```python
from build123d import *

# Parameters (mm, degrees)
F0_R     = 6
F1_DEPTH = 23
F2_SIZE  = 0.5
F3_R     = 1.5
F4_DEPTH = 12.5
F5_R     = 2
F6_DEPTH = 10
F7_SIZE  = 0.25


with BuildPart() as f1:
    # F0 (on Front) → F1 (new body)
    with BuildSketch(Plane.XZ):
        Circle(F0_R)
    extrude(amount=F1_DEPTH)

    # F2
    f2_edges = [f1.edges().sort_by_distance(p)[0] for p in [
        (-6, -23, 0),
        (-6, 0, 0),
    ]]
    chamfer(f2_edges, length=F2_SIZE)

    # F3 (on Right) → F4 (cut, symmetric)
    with BuildSketch(Plane.YZ):
        with Locations((-18, 0)):
            Circle(F3_R)
    extrude(amount=F4_DEPTH, both=True, mode=Mode.SUBTRACT)

    # F5 (on face) → F6 (join)
    with BuildSketch(Plane(origin=(0, 0, 0), x_dir=(-1, 0, 0), z_dir=(0, 1, 0))):
        with Locations((0, -3.3)):
            Circle(F5_R)
    extrude(amount=F6_DEPTH)

    # F7
    f7_edges = [f1.edges().sort_by_distance(p)[0] for p in [
        (2, 10, -3.3),
    ]]
    chamfer(f7_edges, length=F7_SIZE)


solid = f1.part
```
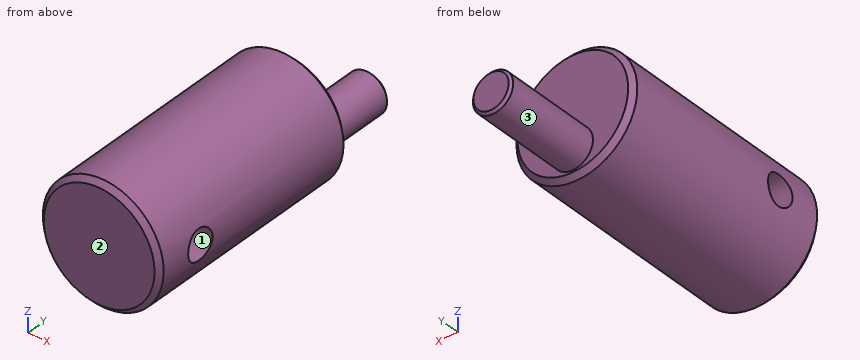
The model under review builds one solid part; all positions refer to its coordinate system, in mm. Face numbers are marked on the shaded views. Round coordinates to 2 decimals unless told otherwise and drop trailing zeros. Order: outer loops, then holes, each group sorted by start corner. A loop starts at its lowest first (then second) coordinate and runs counter-clockwise, first axis right, second up.
Item 1: Add section A-A, the plane z = 0. State the section outline as (x, y) points, and give its area (4 significant figures).
Working result:
outline: (-6, -22.5) - (-5.5, -23) - (5.5, -23) - (6, -22.5) - (6, -19.5) - (-6, -19.5) - close; (-6, -16.5) - (6, -16.5) - (6, -0.5) - (5.5, 0) - (-5.5, 0) - (-6, -0.5) - close
area: 239.5 mm2
Item 2: For pin 1 (2 mm diameter, centred on y = -8.5, z = 4, fed in from +X); pin 2 (2 mm diameter, centred on x = -3, y = -13.5, fed in from +Z); pin 3 (4 mm diameter, centred on y = -18, z = 0, fed in from +X); pin 4 (3 mm diameter, centred on x = -1, z = 3, fed in from +Y), all flat-tipped, find the tip position at first contact; note any pin that passes through.
Working result:
pin 1: stops at x = 5.2
pin 2: stops at z = 5.66
pin 3: stops at x = 6
pin 4: stops at y = 0
Item 3: Add section D-D, the plane y = -18. State the section outline as (x, z) points.
Working result:
outline: (-5.81, -1.5) arc R6 ccw to (5.81, -1.5) - close; (-5.81, 1.5) - (5.81, 1.5) arc R6 ccw to start
Item 4: Add section C-C, the plane y = -10. State the section outline as (x, z) points, and give its area (3 significant figures).
Working result:
outline: circle Ø12 at (0, 0)
area: 113 mm2
Item 5: To check wall thickness, follow probe 1 along Y at (x, z) = (2.75, 0); probe 2 along Z at (x, y) = (-1.75, -18); probe 3 along Y at (x, z) = (-4.25, 0.75). State the ranges of each line that lie inside material, in increasing order.
Working result:
probe 1: y = -23 to -19.5, -16.5 to 0
probe 2: z = -5.74 to -1.5, 1.5 to 5.74
probe 3: y = -23 to -19.3, -16.7 to 0
Item 6: Draft analysis for pull direction Z (two halves, no side actions). For the marked faces 1, 2 and 3, state which applies: released by +Z, released by -Z, zero draft, split by the parting line, or undercut.
Working result:
face 1: undercut
face 2: zero draft
face 3: split by the parting line
Item 7: Add section B-B, the plane x = 0. State the section outline as (y, z) points.
Working result:
outline: (-23, -5.5) - (-22.5, -6) - (-0.5, -6) - (0, -5.5) - (0, -5.3) - (9.75, -5.3) - (10, -5.05) - (10, -1.55) - (9.75, -1.3) - (0, -1.3) - (0, 5.5) - (-0.5, 6) - (-22.5, 6) - (-23, 5.5) - close; hole circle Ø3 at (-18, 0)
